Autodesk Inventor part; units mm, degrees
ref_plane "YZ Plane" through (0, 0, 0) normal (1, 0, 0) x (0, 1, 0)
ref_plane "XZ Plane" through (0, 0, 0) normal (0, 1, 0) x (-1, 0, 0)
ref_plane "XY Plane" through (0, 0, 0) normal (0, 0, 1) x (1, 0, 0)
sketch "Sketch1" plane through (0, 0, 0) normal (0, 0, 1) x (1, 0, 0)
  line L0 (-30, 0) -> (0, 0)
  line L1 (0, 0) -> (0, 50)
  line L2 (0, 50) -> (-30, 50)
  dimension "d0" = 30
  dimension "d1" = 30
  dimension "d2" = 50
contour flange "Contour Flange1" sketch "Sketch1" thickness 3 bend radius 3.9 width 180 along (0, 0, 1) mid plane no both sides no wall seen from (-15, 0, 0) lies toward (0, 1, 0) curves L0 L1 L2
bend "Bend1"
corner "Corner1"
equation "\"d1\" = d0"
equation "\"d3\" = BendReliefWidth"
equation "\"d4\" = BendReliefDepth"
equation "\"d5\" = MinimumRemnant"
equation "\"d6\" = BendRadius"
equation "\"d8\" = BendRadius"
equation "\"d10\" = CornerReliefSize"
equation "\"d11\" = GapSize"
equation "\"d12\" = JacobiRadiusSize"
equation "\"BendReliefWidth\" = Thickness"
equation "\"BendReliefDepth\" = 0.5 * Thickness"
equation "\"CornerReliefSize\" = 4 * Thickness"
equation "\"MinimumRemnant\" = 2 * Thickness"
equation "\"TransitionRadius\" = BendRadius"
equation "\"JacobiRadiusSize\" = BendRadius"
equation "\"GapSize\" = Thickness"
properties part number "Poot"
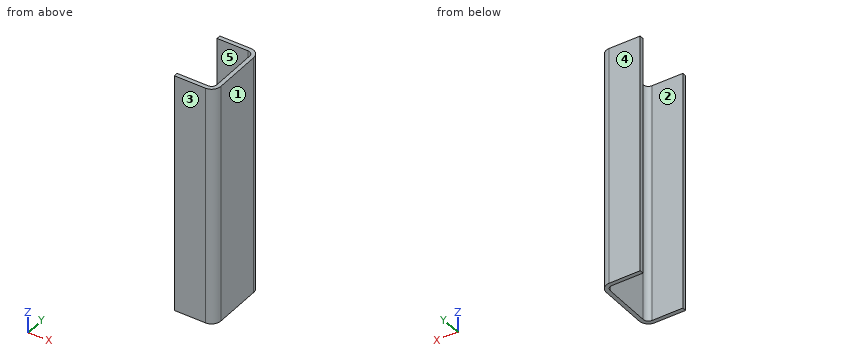
For this review, take the finished solid that the model builds, in its own axes (mm). Face numbers are marked on the shaded views. A direction names the side the tool comes from. Give positions to 0.01 mm unless a question says otherwise; leave off trailing zeros. Loops run counter-clockwise (first coordinate to the right, second up) from the corner with the lowest first, then second, coordinate; pieces in that order, holes last. Notation, with made-up numbers: M 59,33 L 91,33 A34 cw 91,67 Z; hole C 49.25,45 d9. An arc over 180 degrees is marked long. One line per item, written item: value. Start each with the question number.
Q1. Draft analysis for pull direction Y (two halves, no side actions). For the marked faces 3, 4 and 5, state which applies: released by +Y, released by -Y, zero draft, split by the parting line, or undercut.
Q2. Add section C-C (y = 24). Give the boundary of the cut face in (x, z).
Q3. Machinability: for the marked faces 1 and 2, which of the approach directions +Z, -Z, +X, -X, +Y, -Y give a long, thin tool a straight path to every point of the face, cutting with its end or side? Answer none if there is none.
Q4. Add section A-A (x = -14.5). Give the boundary of the cut face in (y, z).
Q5. Clearance check with a flat-ended pin moving along its axis: pin 1 Ø18 at (y, z) = (26.5, 72) entering from -X. State where the tip first meets the part, or that it passes through.
Q6. For L1, parallel to Y at x = -22, z = 111; L2, parallel to X at y = 28.5, z = 145; L3, parallel to Y at x = -4.5, z = 13.5, list the stretches that pass through material, from the lowest coordinate up.
Q7. Add section B-B (z = 148.5). Give the boundary of the cut face in (x, y), and give its area (3 significant figures).
Reply:
1. face 3: released by -Y
1. face 4: released by +Y
1. face 5: undercut
2. outline: M -3,0 L 0,0 L 0,180 L -3,180 Z
3. face 1: +Z, -Z, +X, +Y, -Y
3. face 2: +Z, -Z, -X
4. outline: M 0,0 L 3,0 L 3,180 L 0,180 Z; M 47,0 L 50,0 L 50,180 L 47,180 Z
5. pin 1: x = -3
6. L1: 0 to 3, 47 to 50
6. L2: -3 to 0
6. L3: 0.43 to 3.83, 46.17 to 49.57
7. outline: M -30,0 L -6.9,0 A6.9 ccw 0,6.9 L 0,43.1 A6.9 ccw -6.9,50 L -30,50 L -30,47 L -6.9,47 A3.9 cw -3,43.1 L -3,6.9 A3.9 cw -6.9,3 L -30,3 Z
7. area: 298 mm²
